Autodesk Inventor part; units mm, degrees
ref_plane "YZ Plane" through (0, 0, 0) normal (1, 0, 0) x (0, 1, 0)
ref_plane "XZ Plane" through (0, 0, 0) normal (0, 1, 0) x (-1, 0, 0)
ref_plane "XY Plane" through (0, 0, 0) normal (0, 0, 1) x (1, 0, 0)
sketch "Sketch1" plane through (0, 0, 0) normal (0, 0, 1) x (1, 0, 0)
  line L0 (0, 0) -> (25.4, 0)
  line L1 (25.4, 0) -> (25.4, -25.4)
  line L2 (25.4, -25.4) -> (0, -25.4)
  line L3 (0, -25.4) -> (0, 0)
  dimension "d0" = 25.4
  dimension "d1" = 25.4
extrude "Extrusion1" add sketch "Sketch1" along normal blind 4.8768
sketch "Sketch2" plane through (0, 0, 4.8768) normal (0, 0, 1) x (1, 0, 0)
  line L0 (0, 0) -> (0, -25.4)
  line L1 (0, -12.7) -> (12.7, -12.7)
  line L2 (12.7, -12.7) -> (12.7, -2.921)
  point P0 (5.7852, -5.7852)
  point P1 (2.921, -12.7)
  point P2 (5.7852, -19.6148)
  point P3 (12.7, -22.479)
  point P4 (19.6148, -19.6148)
  point P5 (22.479, -12.7)
  point P6 (19.6148, -5.7852)
  dimension "d4" = 12.7
  dimension "d5" = 9.779
  dimension "d15" = 360
hole "Hole1" at (12.7, -2.921, 4.8768) at (19.6148, -5.7852, 4.8768) at (22.479, -12.7, 4.8768) at (19.6148, -19.6148, 4.8768) at (12.7, -22.479, 4.8768) at (5.7852, -19.6148, 4.8768) at (2.921, -12.7, 4.8768) at (5.7852, -5.7852, 4.8768) direction (0, 0, -1) diameter 2.7178 depth 25.4 tip angle 118
sketch "Sketch3" plane through (0, 0, 4.8768) normal (0, 0, 1) x (1, 0, 0)
  point P0 (0, 0)
properties part number "GlyphtPlateAttachment"
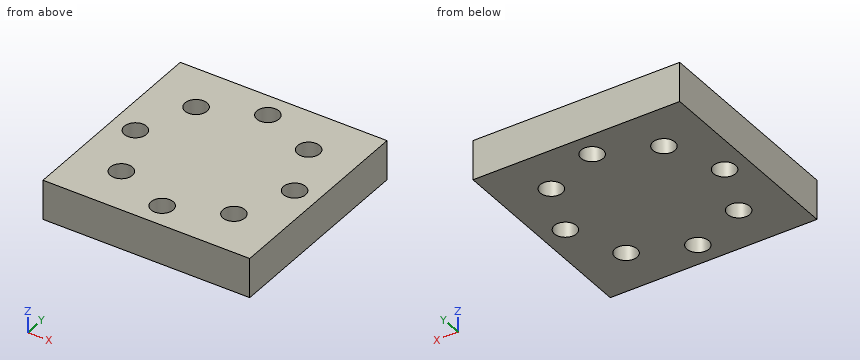
Could you check a few things on this model? Use its own coordinates, in mm. Give positions to 0.01 mm unless a question says otherwise; leave off trailing zeros. Order: outer loops, then holes, each group sorted by start corner. A loop starts at its lowest first (then second) coordinate and runs counter-clockwise, first axis right, second up.
Q1. I'm going to push flat-ended pins straight in: P1, Ø1.6, axis at x = 5.79, y = -19.61, coming from the +Z side; P2, Ø4.5, axis at x = 22.479, y = -12.7, coming from the +Z side. Where does each tip first touch, or does it pass through?
Q2. Suppose I cut it at C-C, the plane z = 3.4. Count the separate pieces of the cut face and the enclosed holes in it, and give its area (3 significant figures).
Q3. If I drill on line 1 along X through (y, z) = (-12.7, 1.6); line 2 along Y through (x, z) = (12.7, 1.4); line 3 along Y through (x, z) = (22.5, 0.2), over which ranges is the centre line in solid material (lowest first)?
Q4. Suppose I cut it at A-A, the plane x = 12.7. Write out the boundary of the cut face in (y, z).
Q5. Suppose I cut it at B-B, the plane y = -12.7. Write out the boundary of the cut face in (x, z), and give its area (3 significant figures).
Solution:
1. P1: passes through
1. P2: stops at z = 4.88
2. separate pieces: 1
2. enclosed holes: 8
2. area: 599 mm2
3. line 1: x = 0 to 1.56, 4.28 to 21.12, 23.84 to 25.4
3. line 2: y = -25.4 to -23.84, -21.12 to -4.28, -1.56 to 0
3. line 3: y = -25.4 to -14.06, -11.34 to 0
4. outline: (-25.4, 0) - (-23.84, 0) - (-23.84, 4.88) - (-25.4, 4.88) - close; (-21.12, 0) - (-4.28, 0) - (-4.28, 4.88) - (-21.12, 4.88) - close; (-1.56, 0) - (0, 0) - (0, 4.88) - (-1.56, 4.88) - close
5. outline: (0, 0) - (1.56, 0) - (1.56, 4.88) - (0, 4.88) - close; (4.28, 0) - (21.12, 0) - (21.12, 4.88) - (4.28, 4.88) - close; (23.84, 0) - (25.4, 0) - (25.4, 4.88) - (23.84, 4.88) - close
5. area: 97.4 mm2
